```python
from build123d import *

# Parameters (mm, degrees)
BOSS_EXTRUDE1_DEPTH = 25
FILLET2_R           = 0.25
FILLET3_R           = 0.5
FILLET5_R           = 0.25
CUT_EXTRUDE2_DEPTH  = 10.448688931


with BuildPart() as part:
    # Sketch1 → Boss-Extrude1 (new body)
    with BuildSketch(Plane.XY):
        with BuildLine():
            Line((-30, 0), (-30, -2))
            ThreePointArc((-30, -2), (0, 7.632365953), (30, -2))
            Line((30, -2), (30, 0))
            ThreePointArc((30, 0), (0, 9.448688831), (-30, 0))
        make_face()
    extrude(amount=BOSS_EXTRUDE1_DEPTH)

    # Fillet2
    fillet2_edges = [part.edges().sort_by_distance(p)[0] for p in [
        (0, 9.448688831, 25),
    ]]
    fillet(fillet2_edges, radius=FILLET2_R)

    # Fillet3
    fillet3_edges = [part.edges().sort_by_distance(p)[0] for p in [
        (0, 7.632365953, 25),
    ]]
    fillet(fillet3_edges, radius=FILLET3_R)

    # Fillet5
    fillet5_edges = [part.edges().sort_by_distance(p)[0] for p in [
        (0, 9.448688831, 0),
        (0, 7.632365953, 0),
    ]]
    fillet(fillet5_edges, radius=FILLET5_R)

    # Sketch6 → Cut-Extrude2 (cut, through all)
    with BuildSketch(Plane(origin=(0, 0, 0), x_dir=(1, 0, 0), z_dir=(0, 1, 0))):
        with BuildLine():
            Line((-15, -8.5), (15, -8.5))
            ThreePointArc((15, -8.5), (19, -12.5), (15, -16.5))
            Line((15, -16.5), (-15, -16.5))
            ThreePointArc((-15, -16.5), (-19, -12.5), (-15, -8.5))
        make_face()
    extrude(amount=CUT_EXTRUDE2_DEPTH, mode=Mode.SUBTRACT)


solid = part.part
```
Design review of the part built by this model. Coordinates are the model's own, in mm. A direction names the side the tool comes from. Give positions to 0.01 mm unless a question says otherwise; leave off trailing zeros. Write each loop counter-clockwise with the first axis right and the second up, starting at its lowest first coordinate (ties: lowest second). Pieces come first, ordered by that corner, then holes. Notation, with made-up numbers: (-5, 11.25) - (22, 11.25) arc R20 ccw to (22, 19.25) - close; hole circle Ø10 at (-11.5, 63). An arc over 180 degrees is marked (long way). Return JSON: item names as keys, results as strings. Group by question number.
(1) Mouldability with a two-part tool opening along X and no side actions: class faces 3 (the flat face through (-30, -1, 12)), 4 (the cylindrical face through (0.447, 9.447, 6.884)), 5 (the cylindrical face through (-19, 5.2, 12.6)) as +X half, -X half, draft (parallel to the pull), parting line (faces both ways), or undercut.
(2) Insertion check: pin 1 (10 mm diameter, centred on x = 17, z = 20.5, fed in from -Y); pin 2 (5 mm diameter, centred on x = 5, z = 6, fed in from -Y); pin 3 (3 mm diameter, centred on y = 8.5, z = 14, fed in from +X). Each pin has a flat end and moves straight along its axis. Give the tip position at first contact, or say it passes through.
(3) We need section A-A, the plane z = 12.5. Give the boundary of the cut face in (x, y), then the cut area to 3 significant figures.
(4) We need section B-B, the plane z = 20.5. Give the boundary of the cut face in (x, y), then the cut area to 3 significant figures.
(5) Machinability: for faces 1 (the cylindrical face through (-0.45, 7.63, 17.59)), 2 (the cylindrical face through (19, 5.2, 12.4)), which of the approach directions +Z, -Z, +X, -X, +Y, -Y give a long, thin tool a straight path to every point of the face, cutting with its end or side? Answer none if there is none.
Reported:
{
 "1": {"face 3": "-X half", "face 4": "parting line", "face 5": "undercut"},
 "2": {"pin 1": "stops at y = 2.7", "pin 2": "stops at y = 7.08", "pin 3": "passes through"},
 "3": {"outline": "(-30, -2) arc R51.53 cw to (-19, 4) - (-19, 5.88) arc R52.35 ccw to (-30, 0) - close; (19, 4) arc R51.53 cw to (30, -2) - (30, 0) arc R52.35 ccw to (19, 5.88) - close", "area": "42.5 mm2"},
 "4": {"outline": "(-30, -2) arc R51.53 cw to (30, -2) - (30, 0) arc R52.35 ccw to (-30, 0) - close", "area": "112 mm2"},
 "5": {"face 1": "+Z, -Z, -Y", "face 2": "+Y, -Y"}
}
